Check sheet for the modelled part. Datum: model origin and axes. Units: mm. Face numbers are marked on the shaded views. A direction names the side the tool comes from. Round coordinates to 2 decimals unless told otherwise and drop trailing zeros. Loops run counter-clockwise (first coordinate to the right, second up) from the corner with the lowest first, then second, coordinate; pieces in that order, holes last. Notation, with made-up numbers: M 74.25,7.5 L 114.25,7.5 A9 cw 114.25,18.5 Z; hole C 19,30.5 d1. An arc over 180 degrees is marked long. One line per question, with ' | ' between items. Start each with the question number.
(1) Section check C-C (x = -34.5). Record the boundary of the cut face in (y, z), and give its area (3 significant figures).
(2) Go/stop test with flat-tipped pins: P1, Ø1.5, axis at y = -35, z = 3.5, coming from the +X side; P2, Ø5.5, axis at x = -11.31, y = -11.31, coming from the +Z side; P3, Ø2, axis at y = -16.5, z = 5, coming from the -X side. Record where each tip stops, or that it passes through.
(3) Draft check along Y on the marked faces 3, 4, 5 and 6. Enter one of: +Y half, -Y half, draft (parallel to the pull), parting line (faces both ways), or undercut.
(4) Section check B-B (x = 23.5). Record the boundary of the cut face in (y, z).
(5) Section check A-A (x = 0). Record the boundary of the cut face in (y, z), and give its area (3 significant figures).
(6) Thickness scan on probe 1 along X at (y, z) = (-8, 6.25); probe 2 along Z at (x, y) = (16, -21); probe 3 along X at (y, z) = (25, 8.5). Record the ranges inside material, lowest first. Write a range as [from, to].
(7) Tool access check on the marked faces 1 and 2. Record the directions out of +Z, -Z, +X, -X, +Y, -Y that give a thin tool (end or side, any length) a straight path to the whole face; none if there is none.
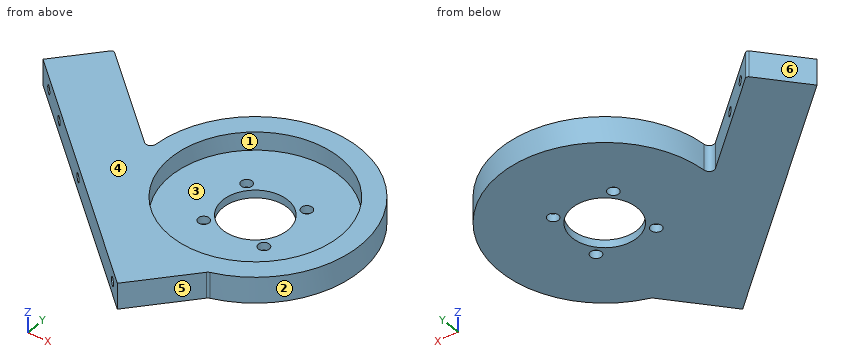
Autodesk Inventor part; units mm, degrees
ref_plane "Work Plane1" through (0, 0, 0) normal (0, 0, 1) x (1, 0, 0)
ref_plane "YZ Plane" through (0, 0, 0) normal (1, 0, 0) x (0, 1, 0)
ref_plane "XZ Plane" through (0, 0, 0) normal (0, 1, 0) x (-1, 0, 0)
ref_plane "Work Plane1" through (0, 0, 0) normal (0, 0, 1) x (1, 0, 0)
sketch "Sketch1" plane through (0, 0, 0) normal (0, 0, 1) x (1, 0, 0)
  arc A0 (-77.068, 33.987) -> (-78.4814, 33.9394) centre (-77.7509, 33.2565) ccw
  line L0 (-78.4814, 33.9394) -> (-92.9244, 18.4887)
  line L1 (-92.9244, 18.4887) -> (-9.2531, -59.7257)
  line L2 (-9.2531, -59.7257) -> (9.7389, -39.4086)
  arc A1 (10.6702, -38.8458) -> (9.7389, -39.4086) centre (11.2, -40.7744) ccw
  arc A2 (10.6702, -38.8458) -> (-40.1013, 3.8394) centre (0, 0) ccw
  line L3 (-43.4579, 2.5689) -> (-77.068, 33.987)
  circle A3 centre (33.3141, 1.123) radius 2.5
  circle A4 centre (1.123, -33.3141) radius 2.5
  circle A5 centre (0, 0) radius 21
  circle A6 centre (-1.123, 33.3141) radius 2.5
  circle A7 centre (-33.3141, -1.123) radius 2.5
  circle A8 centre (0, 0) radius 12.5
  circle A9 centre (0, -16) radius 2
  circle A10 centre (0, 16) radius 2
  circle A11 centre (-16, 0) radius 2
  circle A12 centre (16, 0) radius 2
  circle A13 centre (11.3137, 11.3137) radius 1.6
  circle A14 centre (-11.3137, -11.3137) radius 1.6
  circle A15 centre (-11.3137, 11.3137) radius 1.6
  circle A16 centre (11.3137, -11.3137) radius 1.6
  circle A17 centre (0, 0) radius 20.7
  circle A18 centre (0, 0) radius 40.2846
  line L4 (31.6375, -97.9493) -> (-99.8575, 24.9697)
  arc A19 (-43.4579, 2.5689) -> (-40.1013, 3.8394) centre (-42.0921, 4.03) ccw
  point P0 (0, 0)
  point P1 (-45.0314, -26.2807)
  point P2 (-23.1886, -46.699)
  point P3 (0, 0)
  point P4 (10.6702, -38.8458)
  point P5 (-40.1013, 3.8394)
  point P6 (0, 0)
extrude "Extrusion1" add sketch "Sketch1" along normal blind 10 contours L3 A19 A18 A1 L2 L1 L0 A0 | A2 A18 | A3 | A4 | A5 | A6 | A7 | A9 | A10 | A11 | A12 | A13 | A14 | A15 | A16 | A17
sketch "Sketch2" plane through (-77.068, 33.987, 10) normal (0.6828833, 0.7305275, 0) x (0.7305275, -0.6828833, 0)
  arc A0 (36.818, 70.5) -> (34.818, 72.5) centre (34.818, 70.5) ccw
  line L0 (-3.182, 72.5) -> (34.818, 72.5)
  arc A1 (-3.182, 72.5) -> (-5.182, 70.5) centre (-3.182, 70.5) ccw
  line L1 (-5.182, 2) -> (-5.182, 70.5)
  arc A2 (-5.182, 2) -> (-3.182, 0) centre (-3.182, 2) ccw
  line L2 (34.818, 0) -> (-3.182, 0)
  arc A3 (34.818, 0) -> (36.818, 2) centre (34.818, 2) ccw
  line L3 (36.818, 70.5) -> (36.818, 2)
  circle A4 centre (15.818, 36.25) radius 12.6
  circle A5 centre (31.818, 36.25) radius 2
  arc A6 (31.218, 2.9) -> (31.218, 7.1) centre (31.218, 5) ccw
  line L4 (0.418, 2.9) -> (31.218, 2.9)
  arc A7 (0.418, 7.1) -> (0.418, 2.9) centre (0.418, 5) ccw
  line L5 (31.218, 7.1) -> (0.418, 7.1)
  circle A8 centre (15.818, 20.25) radius 2
  arc A9 (0.418, 69.6) -> (0.418, 65.4) centre (0.418, 67.5) ccw
  line L6 (31.218, 69.6) -> (0.418, 69.6)
  arc A10 (31.218, 65.4) -> (31.218, 69.6) centre (31.218, 67.5) ccw
  line L7 (0.418, 65.4) -> (31.218, 65.4)
  circle A11 centre (15.818, 52.25) radius 2
  circle A12 centre (-0.182, 36.25) radius 2
  circle A13 centre (7.918, 67.5) radius 1.5706
  circle A14 centre (23.718, 67.5) radius 1.5706
  circle A15 centre (28.5459, 23.5221) radius 2
  circle A16 centre (3.09, 23.5221) radius 2
  circle A17 centre (3.09, 48.9779) radius 2
  circle A18 centre (28.5459, 48.9779) radius 2
  point P0 (79.5095, 10)
  point P1 (7.918, 5)
  point P2 (23.718, 5)
hole "Hole1" at (-71.2837, 28.58, 5) at (-59.7414, 17.7904, 5) direction (-0.6828833, -0.7305275, 0) diameter 3.242 end through all
sketch "Sketch9" plane through (0, 0, 10) normal (0, 0, 1) x (1, 0, 0)
  circle A0 centre (0, 0) radius 32.55
  dimension "d44" = 65.1
extrude "Extrusion4" cut sketch "Sketch9" against normal blind 7
sketch "Sketch11" plane through (-9.2531, -59.7257, 0) normal (-0.6828833, -0.7305275, 0) x (0.7305275, -0.6828833, 0)
  circle A0 centre (-60.5521, 5) radius 2.25
  circle A1 centre (-7.5, 5) radius 2.25
  point P0 (-34.026, 0)
hole "Hole7" at (-53.488, -18.3757, 5) at (-14.732, -54.604, 5) direction (0.6828833, 0.7305275, 0) diameter 3.242 depth 15 tip angle 118
sketch "Sketch12" plane through (0, 0, 3) normal (0, 0, 1) x (1, 0, 0)
  circle A0 centre (0, 0) radius 12.5
  circle A1 centre (0, -18) radius 2
  circle A2 centre (0, 18) radius 2
  circle A3 centre (-18, 0) radius 2
  circle A4 centre (18, 0) radius 2
  circle A5 centre (11.3137, 11.3137) radius 1.6
  circle A6 centre (-11.3137, -11.3137) radius 1.6
  circle A7 centre (-11.3137, 11.3137) radius 1.6
  circle A8 centre (11.3137, -11.3137) radius 1.6
  circle A9 centre (0, 0) radius 20.7
  point P0 (0, 0)
hole "Hole8" at (11.3137, 11.3137, 3) at (-11.3137, 11.3137, 3) at (-11.3137, -11.3137, 3) at (11.3137, -11.3137, 3) direction (0, 0, -1) diameter 4.2 depth 12.8 tip angle 118
properties part number "gearboxframv2" material "Aluminum 6061"
The answers:
1) outline: M -36.13,0 L 20.8,0 L 20.8,10 L -36.13,10 Z | area: 569 mm²
2) P1: x = 21.21 | P2: z = 3 | P3: x = -56.56
3) face 3: undercut | face 4: draft | face 5: -Y half | face 6: +Y half
4) outline: M -32.72,0 L 32.72,0 L 32.72,10 L 22.52,10 L 22.52,3 L -22.52,3 L -22.52,10 L -32.72,10 Z
5) outline: M -49.83,0 L -12.5,0 L -12.5,3 L -32.55,3 L -32.55,10 L -49.83,10 Z; M 12.5,0 L 40.28,0 L 40.28,10 L 32.55,10 L 32.55,3 L 12.5,3 Z | area: 370 mm²
6) probe 1: [-64.59, -45.2], [-42.55, -31.55], [31.55, 39.48] | probe 2: [0, 3] | probe 3: [-86.84, -67.45], [-31.59, -20.84], [20.84, 31.59]
7) face 1: +Z | face 2: +Z, -Z
